For this review, use the dimensioned drawing (mm, ordinates from the lowest corner) and the shaded views. A direction names the side the tool comes from. Coordinates: 2 decimals unless noted, no trailing zeros. Write each loop counter-clockwise with the first axis right and the second up, starting at its lowest first coordinate (ties: lowest second). Pieces come first, ordered by that corner, then holes. Notation, with made-up numbers: (62, 22.25) - (80, 22.25) arc R25 cw to (80, 42.25) - close; hole circle Ø4 at (-13, 40). An arc over 180 degrees is marked (long way). Put each result on its own line as item: value.
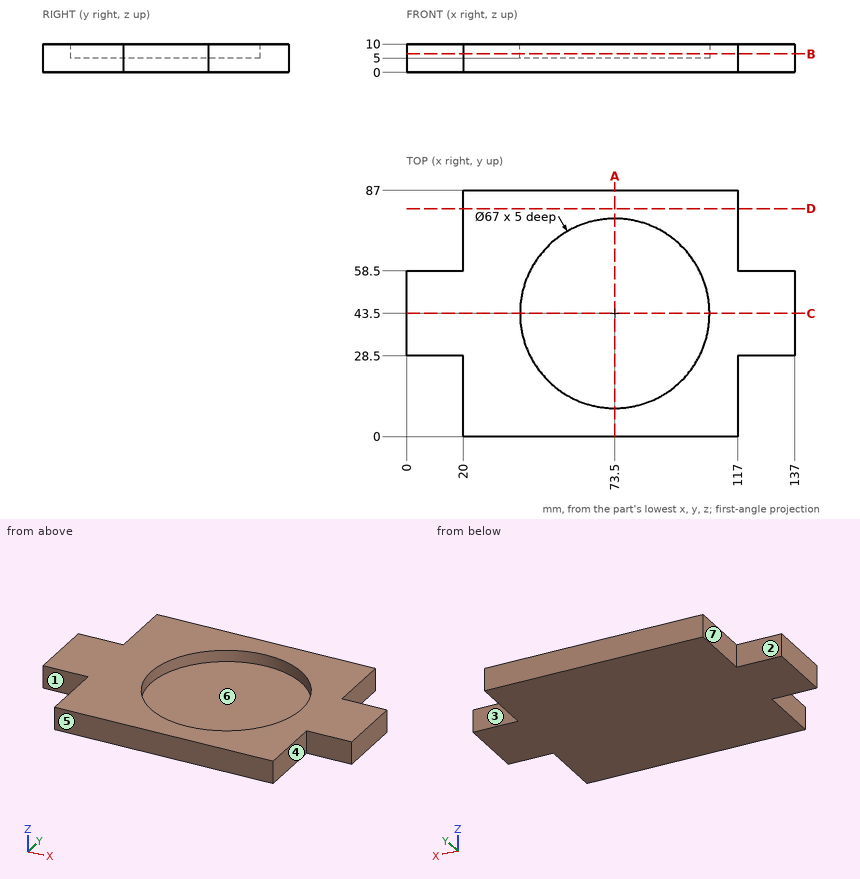
1. Machinability: for the marked faces 1, 2, 3 and 4, which of the approach directions +Z, -Z, +X, -X, +Y, -Y give a long, thin tool a straight path to every point of the face, cutting with its end or side? Answer none if there is none.
Determined:
face 1: +Z, -Z, -X, -Y
face 2: +Z, -Z, -X, +Y
face 3: +Z, -Z, +X, +Y
face 4: +Z, -Z, +X, -Y
2. The part is to be moulded in two halves that separate along Y. For the marked faces 5, 6 and 7, say which applies: +Y half, -Y half, draft (parallel to the pull), parting line (faces both ways), or undercut.
Determined:
face 5: -Y half
face 6: undercut
face 7: draft
3. Consider section A-A on x = 73.5. State the section outline as (y, z) points.
Determined:
outline: (0, 0) - (87, 0) - (87, 10) - (77, 10) - (77, 5) - (10, 5) - (10, 10) - (0, 10) - close
4. To check wall thickness, follow probe 1 along Y at (x, z) = (73.5, 6.95); probe 2 along X at (y, z) = (78, 4.25); probe 3 along Z at (x, y) = (62, 72.5). State the ranges of each line that lie inside material, in increasing order.
Determined:
probe 1: y = 0 to 10, 77 to 87
probe 2: x = 20 to 117
probe 3: z = 0 to 5
5. For pin 1 Ø3 at (x, z) = (14.5, 3) entering from +Y; pin 2 Ø5 at (y, z) = (68.5, 3) entering from +X, all flat-tipped, find the tip position at first contact; note any pin that passes through.
Determined:
pin 1: stops at y = 58.5
pin 2: stops at x = 117
6. Consider section D-D on y = 80.5. State the section outline as (x, z) points, plus the area to 3 significant figures.
Determined:
outline: (20, 0) - (117, 0) - (117, 10) - (20, 10) - close
area: 970 mm^2
7. Consider section B-B on z = 6.5. State the section outline as (x, y) points.
Determined:
outline: (0, 28.5) - (20, 28.5) - (20, 0) - (117, 0) - (117, 28.5) - (137, 28.5) - (137, 58.5) - (117, 58.5) - (117, 87) - (20, 87) - (20, 58.5) - (0, 58.5) - close; hole circle Ø67 at (73.5, 43.5)
8. Consider section C-C on y = 43.5. State the section outline as (x, z) points, plus the area to 4 significant figures.
Determined:
outline: (0, 0) - (137, 0) - (137, 10) - (107, 10) - (107, 5) - (40, 5) - (40, 10) - (0, 10) - close
area: 1,035 mm^2
